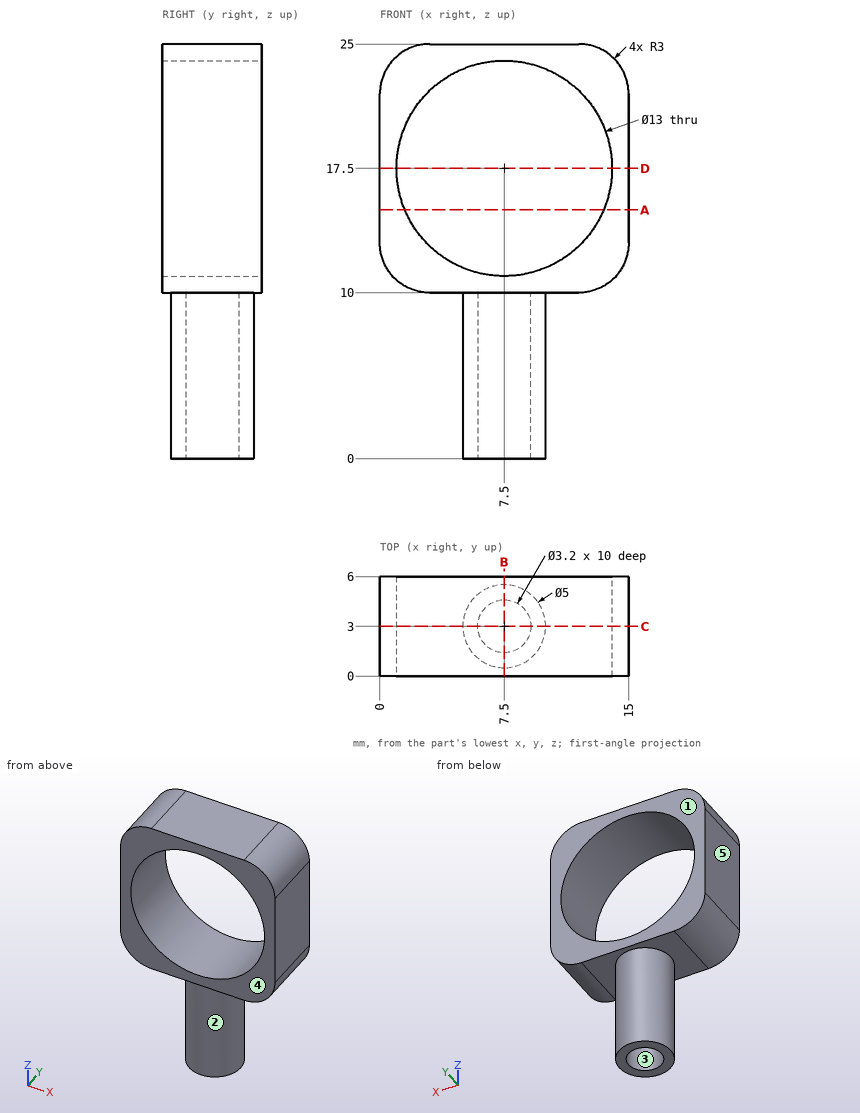
The drawing under review shows one solid part. Ordinate dimensions are in mm from its lowest x, y, z. A direction names the side the tool comes from. Give positions to 0.01 mm unless a question says otherwise; leave off trailing zeros. Loops run counter-clockwise (first coordinate to the right, second up) from the corner with the lowest first, then second, coordinate; pieces in that order, holes last. Notation, with made-up numbers: M -9,8 L 26,8 A22 ccw 26,27 Z; hole C 5.25,-29 d1. An arc over 180 degrees is marked long. Return JSON: item names as keys, results as strings. Group by question number.
Item 1: For probe 1 along Y at (x, z) = (7.5, 7.75); probe 2 along X at (y, z) = (2.3, 14.75); probe 3 along Z at (x, y) = (13.5, 2.25), list the stretches that pass through material, from the lowest coordinate up.
Item 2: We need section A-A (z = 15). Give the boundary of the cut face in (x, y).
Item 3: Insertion check: pin 1 Ø1.5 at (x, y) = (1.5, 2.5) entering from -Z; pin 2 Ø1.5 at (x, y) = (12, 1) entering from -Z. Each pin has a flat end and moves straight along its axis. Give the tip position at first contact, or say it passes through.
Item 4: We need section C-C (y = 3). Give the boundary of the cut face in (x, z).
Item 5: Mouldability with a two-part tool opening along X and no side actions: class the marked faces 3, 4 and 5 as released by +X, released by -X, zero draft, split by the parting line, or undercut.
Item 6: Tool access review of the marked faces 1 and 2: name each direction out of +Z, -Z, +X, -X, +Y, -Y from which nothing blocks a thin tool from reaching the whole face with its end or side.
Item 7: We need section D-D (z = 17.5). Give the boundary of the cut face in (x, y), and give its area (3 significant figures).
Item 8: We need section B-B (x = 7.5). Give the boundary of the cut face in (y, z), and give its area (3 significant figures).
Output:
{
 "1": {"probe 1": "y = 0.5 to 1.4, 4.6 to 5.5", "probe 2": "x = 0 to 1.61, 13.39 to 15", "probe 3": "z = 10.4 to 15, 20 to 24.6"},
 "2": {"outline": "M 0,0 L 1.5,0 L 1.5,6 L 0,6 Z; M 13.5,0 L 15,0 L 15,6 L 13.5,6 Z"},
 "3": {"pin 1": "stops at z = 10.1", "pin 2": "stops at z = 10"},
 "4": {"outline": "M 0,13 A3 ccw 3,10 L 5,10 L 5,0 L 5.9,0 L 5.9,10 L 9.1,10 L 9.1,0 L 10,0 L 10,10 L 12,10 A3 ccw 15,13 L 15,22 A3 ccw 12,25 L 3,25 A3 ccw 0,22 Z; hole C 7.5,17.5 d13"},
 "5": {"face 3": "undercut", "face 4": "zero draft", "face 5": "released by -X"},
 "6": {"face 1": "+Z, -Z, +X, -X, +Y", "face 2": "-Z"},
 "7": {"outline": "M 0,0 L 1,0 L 1,6 L 0,6 Z; M 14,0 L 15,0 L 15,6 L 14,6 Z", "area": "12.0 mm^2"},
 "8": {"outline": "M 0,10 L 0.5,10 L 0.5,0 L 1.4,0 L 1.4,10 L 4.6,10 L 4.6,0 L 5.5,0 L 5.5,10 L 6,10 L 6,11 L 0,11 Z; M 0,24 L 6,24 L 6,25 L 0,25 Z", "area": "30.0 mm^2"}
}
